Input: part model. Units: mm. Frame: model coordinates. A direction names the side the tool comes from. Coordinates: 2 decimals unless noted, no trailing zeros. Write each loop counter-clockwise with the first axis right and the second up, starting at its lowest first coordinate (ties: lowest second). Pieces come first, ordered by that corner, then holes. Notation, with made-up numbers: (58, 0.5) -> (85, 0.5) arc R23 ccw to (85, 17.5) -> close; hole circle Ø2 at (37.5, -13). An arc over 180 degrees is marked (long way). Use one line per item in the form item = value. Start each with the question number.
(1) Pull-direction query (Z, two-part tool) for faces 1 (the face through (116, -12.5, 0)), 2 (the face through (-29, -12, -10)), 3 (the face through (-141.67, -12.68, -0.22)); classes: released by +Z, released by -Z, zero draft, split by the parting line, or undercut.
(2) First-contact query: pin 1 (9 mm diameter, centred on x = -146.67, z = 0, fed in from -Y); pin 2 (5 mm diameter, centred on y = -8, z = -5.5, fed in from +X). Flat tips, straight axial feed; report the tip coordinate or a pass-through.
(3) Cut plane A-A on y = -9.25. Return the cut outline in (x, z).
(4) Set-up query: faces 4 (the face through (115.684, -18.662, 0.74)), 5 (the face through (-94.29, -12.68, 1.83)). Return all of +Z, -Z, +X, -X, +Y, -Y with unobstructed straight access to the full face (end or side cutting, diameter ignored); none if empty.
(5) Cut plane B-B on z = 7.5. Return the cut outline in (x, y).
(6) Ray query, line 1 along Z through (x, y) = (-96.5, -4.75); line 2 along Z through (x, y) = (-26, -9.25); line 3 along Y through (x, z) = (111, 8.75). Return the intervals inside material, ascending.
```python
from build123d import *

# Parameters (mm, degrees)
F0_W     = 50
F0_H     = 10
F0_W_2   = 70
F1_DEPTH = 25
F0_R     = 2.4644634523
F2_DEPTH = 12.5
F3_D     = 10
F4_D     = 10
F5_D     = 6


with BuildPart() as f1:
    # F0 (on Front) → F1 (new body)
    with BuildSketch(Plane.XZ):
        with BuildLine():
            Line((98.3333257594, 10), (-26.6666742406, 10))
            Line((-26.6666742406, 10), (-26.6666742406, 0))
            Line((-26.6666742406, 0), (-26.6666742406, -10))
            Line((-26.6666742406, -10), (98.3333257594, -10))
            ThreePointArc((98.3333257594, -10), (105.4043935713, -7.0710678119), (108.3333257594, 0))
            ThreePointArc((108.3333257594, 0), (105.4043935713, 7.0710678119), (98.3333257594, 10))
        make_face()
        with BuildLine():
            Line((-146.6666742406, 10), (-166.6666742406, 10))
            ThreePointArc((-166.6666742406, 10), (-173.7377420524, 7.0710678119), (-176.6666742406, 0))
            Line((-176.6666742406, 0), (-146.6666742406, 0))
            Line((-146.6666742406, 0), (-146.6666742406, 10))
        make_face()
        with BuildLine():
            Line((-146.6666742406, 0), (-176.6666742406, 0))
            ThreePointArc((-176.6666742406, 0), (-173.7377420524, -7.0710678119), (-166.6666742406, -10))
            Line((-166.6666742406, -10), (-146.6666742406, -10))
            Line((-146.6666742406, -10), (-146.6666742406, 0))
        make_face()
        with Locations((-121.6666742406, -5)):
            Rectangle(F0_W, F0_H)
        with Locations((-61.6666742406, -5)):
            Rectangle(F0_W_2, F0_H)
        with Locations((-121.6666742406, 5)):
            Rectangle(F0_W, F0_H)
        with Locations((-61.6666742406, 5)):
            Rectangle(F0_W_2, F0_H)
    extrude(amount=F1_DEPTH)



with BuildPart() as f1b:
    # F0 (on Front) → F1, piece 2 (new body)
    with BuildSketch(Plane.XZ):
        with Locations((113.3333257594, 0)):
            Circle(F0_R)
    extrude(amount=F1_DEPTH)


with BuildPart() as f1_1:
    add(f1.part)

    add(f1b.part)  # F2 merges F1b
    # F0 (on Front) → F2 (join)
    with BuildSketch(Plane.XZ):
        with BuildLine():
            Line((113.3333257594, 10), (98.3333257594, 10))
            ThreePointArc((98.3333257594, 10), (105.4043935713, 7.0710678119), (108.3333257594, 0))
            ThreePointArc((108.3333257594, 0), (105.4043935713, -7.0710678119), (98.3333257594, -10))
            Line((98.3333257594, -10), (113.3333257594, -10))
            ThreePointArc((113.3333257594, -10), (120.4043935713, -7.0710678119), (123.3333257594, 0))
            ThreePointArc((123.3333257594, 0), (120.4043935713, 7.0710678119), (113.3333257594, 10))
        make_face()
        with Locations((113.3333257594, 0)):
            Circle(F0_R, mode=Mode.SUBTRACT)
    extrude(amount=F2_DEPTH)

    # F3 (through all)
    with Locations(Plane(origin=(0, 0, 0), x_dir=(1, 0, 0), z_dir=(0, 1, 0))):
        with Locations((-146.6666742406, 0)):
            Hole(F3_D / 2)

    # F4 (through all)
    with Locations(Plane(origin=(0, 0, 0), x_dir=(1, 0, 0), z_dir=(0, 1, 0))):
        with Locations((-26.6666742406, 0)):
            Hole(F4_D / 2)

    # F5 (through all)
    with Locations(Plane(origin=(0, 0, 0), x_dir=(1, 0, 0), z_dir=(0, 1, 0))):
        with Locations((-96.6666742406, 0)):
            Hole(F5_D / 2)


solid = f1_1.part
```
Values:
q1.face_1 = zero draft
q1.face_2 = released by -Z
q1.face_3 = undercut
q2.pin_1 = through
q2.pin_2 = 122.87
q3.outline = (-166.67, -10) -> (113.33, -10) arc R10 ccw to (113.33, 10) -> (-166.67, 10) arc R10 ccw to start; hole circle Ø10 at (-146.67, 0); hole circle Ø6 at (-96.67, 0); hole circle Ø10 at (-26.67, 0)
q4.face_4 = -Y
q4.face_5 = +Y, -Y
q5.outline = (-173.28, -25) -> (104.95, -25) -> (104.95, -12.5) -> (119.95, -12.5) -> (119.95, 0) -> (-173.28, 0) -> close
q6.line_1 = -10 to -3, 3 to 10
q6.line_2 = -10 to -4.96, 4.96 to 10
q6.line_3 = -12.5 to 0
